from build123d import *

# Parameters (mm, degrees)
SKETCH_1_R          = 2.15
SKETCH_1_R_2        = 7.125
EXTRUDE_1_DEPTH     = 5
EXTRUDE_START       = -5
SKETCH_2_R          = 13.5
SKETCH_2_R_2        = 9.5
EXTRUDE_2_DEPTH     = 5
CUT_EXTRUDE_START   = -2
SKETCH_3_R          = 4
CUT_EXTRUDE_1_DEPTH = 2
FILLET_START        = 3
FILLET_1_DEPTH      = 3
MOVE_FACE1_BY       = 0.125


with BuildPart() as part:
    # 草图1 → 凸台-拉伸1 (new body)
    with BuildSketch(Plane(origin=(0, 0, 0), x_dir=(0, 0, -1), z_dir=(1, 0, 0))):
        with BuildLine():
            Line((-23.090909091, -3.848365543), (-2.727272727, -9.620913858))
            ThreePointArc((-2.727272727, -9.620913858), (4.253098654, -9.050477989), (9.147283393, -4.040693817))
            Line((9.147283393, -4.040693817), (13.573641697, 5.979653091))
            ThreePointArc((13.573641697, 5.979653091), (13.638118854, 9.867579581), (10.897437667, 12.625984252))
            Line((10.897437667, 12.625984252), (1.979480632, 16.283858268))
            ThreePointArc((1.979480632, 16.283858268), (-9.5, 33.4), (1.979480632, 50.516141732))
            Line((1.979480632, 50.516141732), (10.897437667, 54.174015748))
            ThreePointArc((10.897437667, 54.174015748), (13.545928712, 60.881953925), (6.736898846, 63.258516924))
            Line((6.736898846, 63.258516924), (-8.810480924, 55.366813539))
            ThreePointArc((-8.810480924, 55.366813539), (-10.081211961, 54.350712224), (-10.842152772, 52.912592502))
            Line((-10.842152772, 52.912592502), (-25.842152772, 1.112592502))
            ThreePointArc((-25.842152772, 1.112592502), (-25.498078189, -1.939961078), (-23.090909091, -3.848365543))
        make_face()
        with Locations((9, 58.8)):
            Circle(SKETCH_1_R, mode=Mode.SUBTRACT)
        with Locations((-22, 0)):
            Circle(SKETCH_1_R, mode=Mode.SUBTRACT)
        with Locations((-7, 51.8)):
            Circle(SKETCH_1_R, mode=Mode.SUBTRACT)
        with Locations((9, 8)):
            Circle(SKETCH_1_R, mode=Mode.SUBTRACT)
        Circle(SKETCH_1_R_2, mode=Mode.SUBTRACT)
    extrude(amount=EXTRUDE_1_DEPTH)

    # 草图2 → 凸台-拉伸2 (add)
    # profile 1 of 2: a face of its own
    with BuildSketch(Plane(origin=(5, 0, 0), x_dir=(0, 0, -1), z_dir=(1, 0, 0)).offset(EXTRUDE_START)):
        with BuildLine():
            Line((21.721644442, 37.917716535), (13.711720164, 60.473228346))
            ThreePointArc((13.711720164, 60.473228346), (13.565113542, 56.760456337), (10.897437667, 54.174015748))
            Line((10.897437667, 54.174015748), (1.979480632, 50.516141732))
            ThreePointArc((1.979480632, 50.516141732), (-9.5, 33.4), (1.979480632, 16.283858268))
            Line((1.979480632, 16.283858268), (10.897437667, 12.625984252))
            ThreePointArc((10.897437667, 12.625984252), (13.565113542, 10.039543663), (13.711720164, 6.326771654))
            Line((13.711720164, 6.326771654), (21.721644442, 28.882283465))
            ThreePointArc((21.721644442, 28.882283465), (-4.5, 33.4), (21.721644442, 37.917716535))
        make_face()
    # profile 2 of 2: a face of its own
    with BuildSketch(Plane(origin=(5, 0, 0), x_dir=(0, 0, -1), z_dir=(1, 0, 0)).offset(EXTRUDE_START)):
        with Locations((9, 33.4)):
            Circle(SKETCH_2_R)
        with Locations((9, 33.4)):
            Circle(SKETCH_2_R_2, mode=Mode.SUBTRACT)
    extrude(amount=EXTRUDE_2_DEPTH)

    # 草图3 → 切除-拉伸1 (cut)
    with BuildSketch(Plane(origin=(5, 0, 0), x_dir=(0, 0, -1), z_dir=(1, 0, 0)).offset(CUT_EXTRUDE_START)):
        with Locations((-7, 51.8)):
            Circle(SKETCH_3_R)
        with Locations((9, 8)):
            Circle(SKETCH_3_R)
    extrude(amount=CUT_EXTRUDE_1_DEPTH, mode=Mode.SUBTRACT)

    # 圆角1: read off the stored shape, not the designer's step
    # 圆角1 outline → 圆角1 (cut)
    with BuildSketch(Plane.YZ.offset(FILLET_START)):
        with BuildLine():
            ThreePointArc((49.070439729, 11.954745274), (49.775814705, 11.174989574), (49.393833283, 10.195365665))
            ThreePointArc((49.393833283, 10.195365665), (51.07687003, 10.934092404), (52.912592502, 10.842152772))
            Line((52.912592502, 10.842152772), (49.070439729, 11.954745274))
        make_face()
        with BuildLine():
            ThreePointArc((55.388472863, 5.232837723), (56.279537114, 5.791028828), (57.177294463, 5.243667384))
            Line((57.177294463, 5.243667384), (55.366813539, 8.810480924))
            ThreePointArc((55.366813539, 8.810480924), (55.799926698, 7.02421586), (55.388472863, 5.232837723))
        make_face()
    extrude(amount=FILLET_1_DEPTH, mode=Mode.SUBTRACT)

    # Move Face1: a curved face moved inward by 0.125
    add(Solid.thicken(part.faces().sort_by_distance((2.5, 33.4, 0.5))[0], -MOVE_FACE1_BY), mode=Mode.SUBTRACT)


solid = part.part
Read the model definition and answer for the solid it produces. Units are mm, in the model's axes. A direction names the side the tool comes from. Give positions to 0.01 mm unless a question says otherwise; leave off trailing zeros. Write each loop counter-clockwise with the first axis right and the second up, starting at its lowest first coordinate (ties: lowest second). Pieces come first, ordered by that corner, then holes. Notation, with made-up numbers: (-9, 64.5) - (2, 64.5) arc R24 cw to (2, 88.5) - close; hole circle Ø8 at (59.5, -20). An arc over 180 degrees is marked (long way). Use CSV: the item, a comma, the result in double quotes. Start each with the question number.
(1) Consider line 1 along Z through (x, y) = (0.7, -1); line 2 along Y through (x, z) = (2.4, -4); line 3 along Y through (x, z) = (1, -6). Determine where each line is inside the solid, lowest interval first.
(2) Determine the mould class of faces 5 (the cylindrical face through (1.48, 49.7, 7.47)), 6 (the flat face through (2.465, -6.694, 13.052)), 7 (the flat face through (5, 27, 2)) for opening direction Y: +Y half, -Y half, draft (parallel to the pull), parting line (faces both ways), or undercut.
(3) Find section C-C (z = 22). Give the vertices of the cut face in (x, y).
(4) Find section D-D (y = 0). Give the vertices of the cut face in (x, z) (3 decimals).
(5) For faces 1 (the cylindrical face through (2.5, 39.9, -1.9)), 2 (the cylindrical face through (3.986, 49.773, 11.19)), 3 (the cylindrical face through (4, 5.6, -5.8)), 4 (the cylindrical face through (3.99, 56.26, 5.79)), determine the directions among +Z, -Z, +X, -X, +Y, -Y from which every point of the face is accessible in a straight line to the end or side of a thin tool.
(6) Find section B-B (y = 39). Give the vertices of the cut face in (x, z).
(7) Given P1, Ø5, axis at y = 58.8, z = -9, coming from the +X side; P2, Ø1, axis at x = 2.5, y = 49.5, coming from the +Z side; P3, Ø2.5, axis at y = 8, z = -9, coming from the +X side; P4, Ø1, axis at x = 1.5, z = 8, coming from the -Y side, each flat-ended and moving along its own axis, determine where each tip first touches the part or whether it passes through.
(8) Find section A-A (x = 2). Give the vertices of the cut face in (y, z) (3 decimals).
Findings below:
1,line 1,"-10.49 to -7.05, 7.05 to 20.1, 23.9 to 25.87"
1,line 2,"-9.17 to -5.9, 5.9 to 25.18, 41.62 to 61.87"
1,line 3,"-8 to -3.84, 3.84 to 24.25, 42.55 to 62.88"
2,face 5,"undercut"
2,face 6,"-Y half"
2,face 7,"draft"
3,outline,"(0, -4.16) - (5, -4.16) - (5, -2.15) - (0, -2.15) - close; (0, 2.15) - (5, 2.15) - (5, 14.38) - (0, 14.38) - close"
4,outline,"(0, -10.932) - (5, -10.932) - (5, -7.125) - (0, -7.125) - close; (0, 7.125) - (5, 7.125) - (5, 19.85) - (0, 19.85) - close; (0, 24.15) - (5, 24.15) - (5, 26) - (0, 26) - close"
5,face 1,"+X, -X"
5,face 2,"+X, +Y"
5,face 3,"+X"
5,face 4,"+Z, +X"
6,outline,"(0, -21.34) - (5, -21.34) - (5, -16.83) - (0, -16.83) - close; (0, -1.17) - (5, -1.17) - (5, 14.87) - (0, 14.87) - close"
7,P1,"x = 5"
7,P2,"z = 11.98"
7,P3,"through"
7,P4,"y = -8.27"
8,outline,"(-9.621, 2.727) arc R10 ccw to (-4.041, -9.147) - (5.98, -13.574) arc R5 ccw to (6.327, -13.712) - (28.882, -21.722) arc R13.5 ccw to (37.918, -21.722) - (60.473, -13.712) arc R5 ccw to (63.259, -6.737) - (55.367, 8.81) arc R4 ccw to (52.913, 10.842) - (1.113, 25.842) arc R4 ccw to (-3.848, 23.091) - close; hole circle Ø14.25 at (0, 0); hole circle Ø4.3 at (0, 22); hole circle Ø4.3 at (8, -9); hole circle Ø19.25 at (33.4, -9); hole circle Ø4.3 at (51.8, 7); hole circle Ø4.3 at (58.8, -9)"
